Answer from the drawing. Dimensions are ordinates in mm from the lowest x, y and z of the part. A direction names the side the tool comes from. Coordinates: 2 decimals unless noted, no trailing zeros. Loops run counter-clockwise (first coordinate to the right, second up) from the corner with the lowest first, then second, coordinate; pieces in that order, holes last. Notation, with made-up numbers: (55, 64) -> (63, 64) arc R29 ccw to (63, 92) -> close; hole circle Ø2 at (80.5, 42.25). An arc over 180 degrees is marked (long way). Use a Markdown table: item, result.
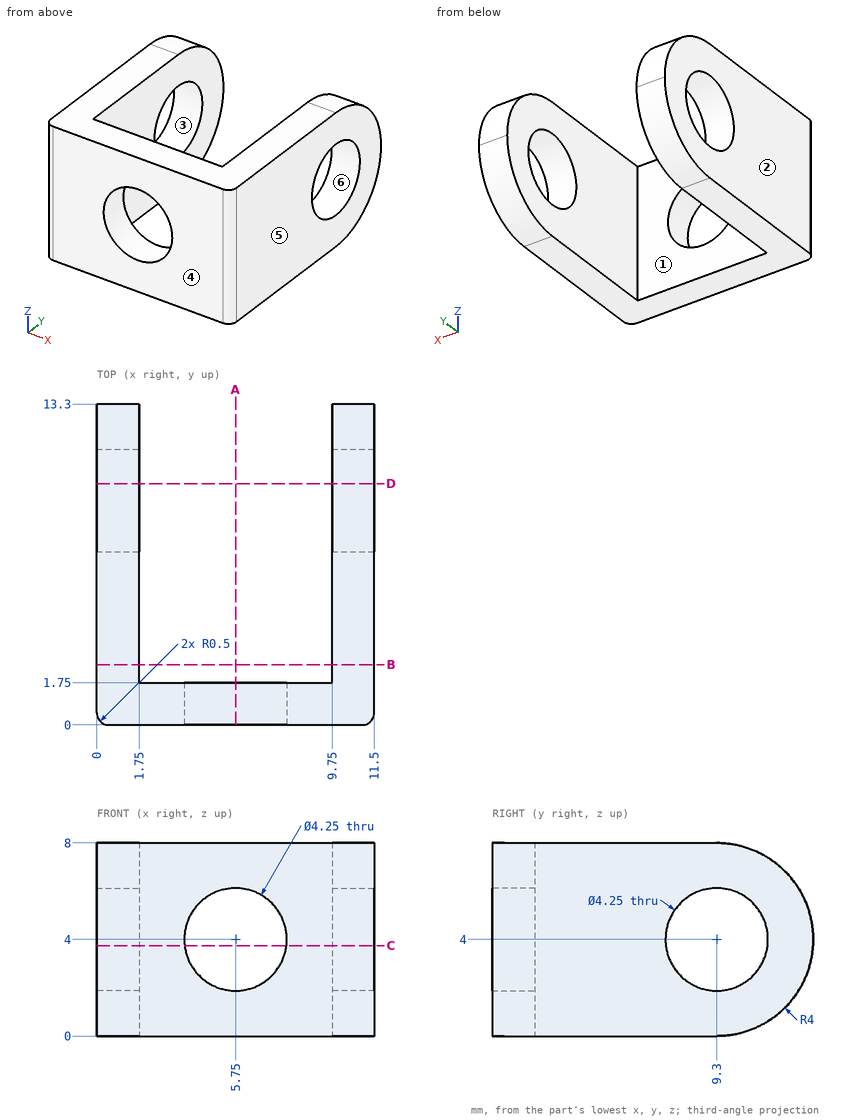
Q1. Section A-A on x = 5.75 is taken. Determine the outline of the cut face in (y, z) (3 decimals).
Solved:
| item | result |
|---|---|
| outline | (0, 0) -> (1.75, 0) -> (1.75, 1.875) -> (0, 1.875) -> close; (0, 6.125) -> (1.75, 6.125) -> (1.75, 8) -> (0, 8) -> close |
Q2. For the marked faces 1 and 2, determine the directions among +Z, -Z, +X, -X, +Y, -Y from which every point of the face is accessible in a straight line to the end or side of a thin tool.
Solved:
| item | result |
|---|---|
| face 1 | +Z, -Z, +Y |
| face 2 | +Z, -Z, -X, +Y, -Y |
Q3. Consider line 1 (X direction, y = 7, z = 0.5); line 2 (Y direction, x = 9.5, z = 1.25); line 3 (Z direction, x = 4.5, y = 1.5). Determine where each line is inside the solid, lowest interval first. Write a range as [from, to].
Solved:
| item | result |
|---|---|
| line 1 | [0, 1.75], [9.75, 11.5] |
| line 2 | [0, 1.75] |
| line 3 | [0, 2.28], [5.72, 8] |
Q4. Section C-C on z = 3.75 is taken. Determine the outline of the cut face in (x, y).
Solved:
| item | result |
|---|---|
| outline | (0, 0.5) arc R0.5 ccw to (0.5, 0) -> (3.64, 0) -> (3.64, 1.75) -> (1.75, 1.75) -> (1.75, 7.19) -> (0, 7.19) -> close; (0, 11.41) -> (1.75, 11.41) -> (1.75, 13.29) -> (0, 13.29) -> close; (7.86, 0) -> (11, 0) arc R0.5 ccw to (11.5, 0.5) -> (11.5, 7.19) -> (9.75, 7.19) -> (9.75, 1.75) -> (7.86, 1.75) -> close; (9.75, 11.41) -> (11.5, 11.41) -> (11.5, 13.29) -> (9.75, 13.29) -> close |
Q5. Section B-B on y = 2.5 is taken. Determine the outline of the cut face in (x, z).
Solved:
| item | result |
|---|---|
| outline | (0, 0) -> (1.75, 0) -> (1.75, 8) -> (0, 8) -> close; (9.75, 0) -> (11.5, 0) -> (11.5, 8) -> (9.75, 8) -> close |
Q6. Section D-D on y = 10 is taken. Determine the outline of the cut face in (x, z), and give its area (3 significant figures).
Solved:
| item | result |
|---|---|
| outline | (0, 0.06) -> (1.75, 0.06) -> (1.75, 1.99) -> (0, 1.99) -> close; (0, 6.01) -> (1.75, 6.01) -> (1.75, 7.94) -> (0, 7.94) -> close; (9.75, 0.06) -> (11.5, 0.06) -> (11.5, 1.99) -> (9.75, 1.99) -> close; (9.75, 6.01) -> (11.5, 6.01) -> (11.5, 7.94) -> (9.75, 7.94) -> close |
| area | 13.5 mm² |
Q7. Given pin 1 Ø4 at (x, z) = (7, 4.5) entering from +Y, flat-ended and moving along its own axis, determine where the tip first touches the part or whether it passes through.
Solved:
| item | result |
|---|---|
| pin 1 | y = 1.75 |
Q8. Determine the mould class of the marked faces 3, 4, 5 and 6 for opening direction Y: pulls with the +Y half, pulls with the -Y half, needs draft (parallel to the pull), parting line crosses it, or undercut.
Solved:
| item | result |
|---|---|
| face 3 | undercut |
| face 4 | pulls with the -Y half |
| face 5 | needs draft |
| face 6 | undercut |
